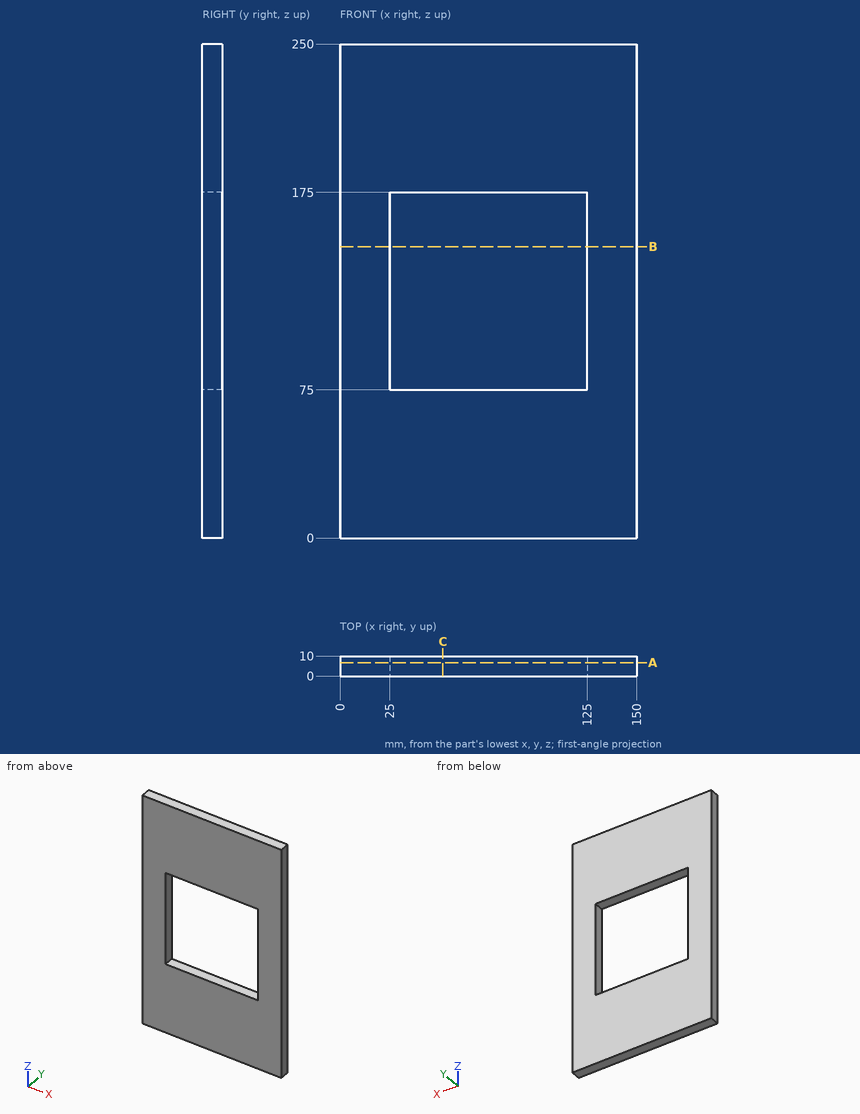
Study the drawing (mm; zero at the part's minimum x, y, z) and answer. Give positions to 0.01 mm unless a question says otherwise; leave off trailing zeros. Write each loop counter-clockwise with the first axis right and the second up, starting at its lowest first coordinate (ties: lowest second). Pieces come first, ordered by that corner, then holes.
(1) The part is cut by section B-B on z = 147.5. Write down the section's boundary in (x, y).
Final values:
outline: (0, 0) - (25, 0) - (25, 10) - (0, 10) - close; (125, 0) - (150, 0) - (150, 10) - (125, 10) - close
(2) The part is cut by section C-C on x = 52. Write down the section's boundary in (y, z).
Final values:
outline: (0, 0) - (10, 0) - (10, 75) - (0, 75) - close; (0, 175) - (10, 175) - (10, 250) - (0, 250) - close
(3) The part is cut by section A-A on y = 6.75. Write down the section's boundary in (x, z), plus the area to 3 significant figures.
Final values:
outline: (0, 0) - (150, 0) - (150, 250) - (0, 250) - close; hole (25, 75) - (125, 75) - (125, 175) - (25, 175) - close
area: 27,500 mm2
(4) Straight lines are drawn through the part: line 1 (Z direction, x = 52, y = 3.75); line 2 (X direction, y = 4.25, z = 154.5). For each, find the intervals that lie inside material, in ascending order.
Final values:
line 1: z = 0 to 75, 175 to 250
line 2: x = 0 to 25, 125 to 150
